from build123d import *

# Parameters (mm, degrees)
F0_R         = 30
F1_DEPTH     = 5
F2_T4_ANGLE  = 130.4484876855
F2_T9_ANGLE  = 130.4484876855
F2_T14_ANGLE = 130.4484876855
F2_T19_ANGLE = 130.4484876855
F2_T24_ANGLE = 130.4484876855
F2_T29_ANGLE = 130.4484876855
F2_T34_ANGLE = 130.4484876855
F2_T39_ANGLE = 130.4484876855
F2_T44_ANGLE = 130.4484876855
F2_T49_ANGLE = 130.4484876855


# Not quite as in the source:
# - a fillet or chamfer that OpenCascade refuses, or shapes differently, is made with other operations: its cross-section is extruded or revolved along the edge and cut away or added


with BuildPart() as f1:
    # F0 (on Top) → F1 (new body)
    with BuildSketch(Plane.XY):
        with BuildLine():
            Line((-40, 12.9967878493), (-24.72135955, 34.0260323341))
            ThreePointArc((-24.72135955, 34.0260323341), (-45.1291822893, 39.7035462239), (-64.2705098312, 30.6303454181))
            Line((-64.2705098312, 30.6303454181), (-40, 12.9967878493))
        make_face()
        Polygon((40, -12.9967878493), (40, 12.9967878493), (24.72135955, 34.0260323341), (0, 42.0584889695), (-24.72135955, 34.0260323341), (-40, 12.9967878493), (-40, -12.9967878493), (-24.72135955, -34.0260323341), (0, -42.0584889695), (24.72135955, -34.0260323341), align=None)
        Circle(F0_R, mode=Mode.SUBTRACT)
        with BuildLine():
            Line((-24.72135955, 34.0260323341), (0, 42.0584889695))
            ThreePointArc((0, 42.0584889695), (-13.1731164802, 58.6471114297), (-33.9918693812, 62.5577278229))
            Line((-33.9918693812, 62.5577278229), (-24.72135955, 34.0260323341))
        make_face()
        with BuildLine():
            Line((0, 42.0584889695), (24.72135955, 34.0260323341))
            ThreePointArc((24.72135955, 34.0260323341), (23.8146320866, 55.1894734115), (9.2705098312, 70.5901844584))
            Line((9.2705098312, 70.5901844584), (0, 42.0584889695))
        make_face()
        with BuildLine():
            Line((24.72135955, 34.0260323341), (40, 12.9967878493))
            ThreePointArc((40, 12.9967878493), (51.7060006259, 30.6513323712), (48.9918693812, 51.6595899029))
            Line((48.9918693812, 51.6595899029), (24.72135955, 34.0260323341))
        make_face()
        with BuildLine():
            Line((70, 12.9967878493), (40, 12.9967878493))
            Line((40, 12.9967878493), (40, -12.9967878493))
            ThreePointArc((40, -12.9967878493), (59.8474343484, -5.5945758344), (70, 12.9967878493))
        make_face()
        with BuildLine():
            Line((64.2705098312, -30.6303454181), (40, -12.9967878493))
            Line((40, -12.9967878493), (24.72135955, -34.0260323341))
            ThreePointArc((24.72135955, -34.0260323341), (45.1291822893, -39.7035462239), (64.2705098312, -30.6303454181))
        make_face()
        with BuildLine():
            Line((33.9918693812, -62.5577278229), (24.72135955, -34.0260323341))
            Line((24.72135955, -34.0260323341), (0, -42.0584889695))
            ThreePointArc((0, -42.0584889695), (13.1731164802, -58.6471114297), (33.9918693812, -62.5577278229))
        make_face()
        with BuildLine():
            Line((-9.2705098312, -70.5901844584), (0, -42.0584889695))
            Line((0, -42.0584889695), (-24.72135955, -34.0260323341))
            ThreePointArc((-24.72135955, -34.0260323341), (-23.8146320866, -55.1894734115), (-9.2705098312, -70.5901844584))
        make_face()
        with BuildLine():
            Line((-48.9918693812, -51.6595899029), (-24.72135955, -34.0260323341))
            Line((-24.72135955, -34.0260323341), (-40, -12.9967878493))
            ThreePointArc((-40, -12.9967878493), (-51.7060006259, -30.6513323712), (-48.9918693812, -51.6595899029))
        make_face()
        with BuildLine():
            Line((-40, -12.9967878493), (-40, 12.9967878493))
            ThreePointArc((-40, 12.9967878493), (-59.8474343484, 5.5945758344), (-70, -12.9967878493))
            Line((-70, -12.9967878493), (-40, -12.9967878493))
        make_face()
    extrude(amount=F1_DEPTH)

    # F2: chamfer of 5 on 10 edges, made by hand


with BuildPart() as f2_tool2:
    # F2_s3 → F2_t4 (revolve)
    with BuildSketch(Plane(origin=(-19.7412033785, -21.6824721062, 0), x_dir=(0, 0, 1), z_dir=(0.6732302342, 0.7394329258, 0))):
        Polygon((0, 1.9388571331), (5, 6.9388571331), (5, 1.9388571331), align=None)
    revolve(axis=Axis((4.103379024, -43.3922083566, 5), (0, 0, 1)), revolution_arc=F2_T4_ANGLE)

    split(bisect_by=Plane(origin=(7.639320225, -10.5146222424, 0), x_dir=(0, 0, 1), z_dir=(0.5877852523, -0.8090169944, 0)), keep=Keep.TOP)


with BuildPart() as f1_1:
    add(f1.part)

    # F2_t1: cut F2_tool2
    add(f2_tool2.part, mode=Mode.SUBTRACT)


with BuildPart() as f2_tool7:
    # F2_s8 → F2_t9 (revolve)
    with BuildSketch(Plane(origin=(-28.7156063599, -5.9379002056, 0), x_dir=(0, 0, 1), z_dir=(0.9792824694, 0.2024990002, 0))):
        Polygon((0, 1.9388571331), (5, 6.9388571331), (5, 1.9388571331), align=None)
    revolve(axis=Axis((-22.1855967717, -37.5169396588, 5), (0, 0, 1)), revolution_arc=F2_T9_ANGLE)

    split(bisect_by=Plane.XZ.offset(12.9967878493), keep=Keep.TOP)


with BuildPart() as f1_2:
    add(f1_1.part)

    # F2_t6: cut F2_tool7
    add(f2_tool7.part, mode=Mode.SUBTRACT)


with BuildPart() as f2_tool12:
    # F2_s13 → F2_t14 (revolve)
    with BuildSketch(Plane(origin=(-26.7216237194, 12.0747477518, 0), x_dir=(0, 0, 1), z_dir=(0.911282086, -0.4117826609, 0))):
        Polygon((0, 1.9388571331), (5, 6.9388571331), (5, 1.9388571331), align=None)
    revolve(axis=Axis((-40.0004286612, -17.3114751652, 5), (0, 0, 1)), revolution_arc=F2_T14_ANGLE)

    split(bisect_by=Plane(origin=(-7.639320225, -10.5146222424, 0), x_dir=(0, 0, 1), z_dir=(-0.5877852523, -0.8090169944, 0)), keep=Keep.TOP)


with BuildPart() as f1_3:
    add(f1_2.part)

    # F2_t11: cut F2_tool12
    add(f2_tool12.part, mode=Mode.SUBTRACT)


with BuildPart() as f2_tool17:
    # F2_s18 → F2_t19 (revolve)
    with BuildSketch(Plane(origin=(-14.5208890526, 25.4752524735, 0), x_dir=(0, 0, 1), z_dir=(0.495202919, -0.8687773415, 0))):
        Polygon((0, 1.9388571331), (5, 6.9388571331), (5, 1.9388571331), align=None)
    revolve(axis=Axis((-42.5364563668, 9.5063844461, 5), (0, 0, 1)), revolution_arc=F2_T19_ANGLE)

    split(bisect_by=Plane(origin=(-12.360679775, -4.0162283177, 0), x_dir=(0, 0, 1), z_dir=(-0.9510565163, -0.3090169944, 0)), keep=Keep.TOP)


with BuildPart() as f1_4:
    add(f1_3.part)

    # F2_t16: cut F2_tool17
    add(f2_tool17.part, mode=Mode.SUBTRACT)


with BuildPart() as f2_tool22:
    # F2_s23 → F2_t24 (revolve)
    with BuildSketch(Plane(origin=(3.2263316853, 29.1450766224, 0), x_dir=(0, 0, 1), z_dir=(-0.1100269317, -0.9939286062, 0))):
        Polygon((0, 1.9388571331), (5, 6.9388571331), (5, 1.9388571331), align=None)
    revolve(axis=Axis((-28.8250035012, 32.6931283091, 5), (0, 0, 1)), revolution_arc=F2_T24_ANGLE)

    split(bisect_by=Plane(origin=(-12.360679775, 4.0162283177, 0), x_dir=(0, 0, 1), z_dir=(-0.9510565163, 0.3090169944, 0)), keep=Keep.TOP)


with BuildPart() as f1_5:
    add(f1_4.part)

    # F2_t21: cut F2_tool22
    add(f2_tool22.part, mode=Mode.SUBTRACT)


with BuildPart() as f2_tool27:
    # F2_s28 → F2_t29 (revolve)
    with BuildSketch(Plane(origin=(19.7412033785, 21.6824721062, 0), x_dir=(0, 0, 1), z_dir=(-0.6732302342, -0.7394329258, 0))):
        Polygon((0, 1.9388571331), (5, 6.9388571331), (5, 1.9388571331), align=None)
    revolve(axis=Axis((-4.103379024, 43.3922083566, 5), (0, 0, 1)), revolution_arc=F2_T29_ANGLE)

    split(bisect_by=Plane(origin=(-7.639320225, 10.5146222424, 0), x_dir=(0, 0, 1), z_dir=(-0.5877852523, 0.8090169944, 0)), keep=Keep.TOP)


with BuildPart() as f1_6:
    add(f1_5.part)

    # F2_t26: cut F2_tool27
    add(f2_tool27.part, mode=Mode.SUBTRACT)


with BuildPart() as f2_tool32:
    # F2_s33 → F2_t34 (revolve)
    with BuildSketch(Plane(origin=(28.7156063599, 5.9379002056, 0), x_dir=(0, 0, 1), z_dir=(-0.9792824694, -0.2024990002, 0))):
        Polygon((0, 1.9388571331), (5, 6.9388571331), (5, 1.9388571331), align=None)
    revolve(axis=Axis((22.1855967717, 37.5169396588, 5), (0, 0, 1)), revolution_arc=F2_T34_ANGLE)

    split(bisect_by=Plane.XZ.offset(-12.9967878493), keep=Keep.BOTTOM)


with BuildPart() as f1_7:
    add(f1_6.part)

    # F2_t31: cut F2_tool32
    add(f2_tool32.part, mode=Mode.SUBTRACT)


with BuildPart() as f2_tool37:
    # F2_s38 → F2_t39 (revolve)
    with BuildSketch(Plane(origin=(26.7216237194, -12.0747477518, 0), x_dir=(0, 0, 1), z_dir=(-0.911282086, 0.4117826609, 0))):
        Polygon((0, 1.9388571331), (5, 6.9388571331), (5, 1.9388571331), align=None)
    revolve(axis=Axis((40.0004286612, 17.3114751652, 5), (0, 0, 1)), revolution_arc=F2_T39_ANGLE)

    split(bisect_by=Plane(origin=(7.639320225, 10.5146222424, 0), x_dir=(0, 0, 1), z_dir=(0.5877852523, 0.8090169944, 0)), keep=Keep.TOP)


with BuildPart() as f1_8:
    add(f1_7.part)

    # F2_t36: cut F2_tool37
    add(f2_tool37.part, mode=Mode.SUBTRACT)


with BuildPart() as f2_tool42:
    # F2_s43 → F2_t44 (revolve)
    with BuildSketch(Plane(origin=(14.5208890526, -25.4752524735, 0), x_dir=(0, 0, 1), z_dir=(-0.495202919, 0.8687773415, 0))):
        Polygon((0, 1.9388571331), (5, 6.9388571331), (5, 1.9388571331), align=None)
    revolve(axis=Axis((42.5364563668, -9.5063844461, 5), (0, 0, 1)), revolution_arc=F2_T44_ANGLE)

    split(bisect_by=Plane(origin=(12.360679775, 4.0162283177, 0), x_dir=(0, 0, 1), z_dir=(0.9510565163, 0.3090169944, 0)), keep=Keep.TOP)


with BuildPart() as f1_9:
    add(f1_8.part)

    # F2_t41: cut F2_tool42
    add(f2_tool42.part, mode=Mode.SUBTRACT)


with BuildPart() as f2_tool47:
    # F2_s48 → F2_t49 (revolve)
    with BuildSketch(Plane(origin=(-3.2263316853, -29.1450766224, 0), x_dir=(0, 0, 1), z_dir=(0.1100269317, 0.9939286062, 0))):
        Polygon((0, 1.9388571331), (5, 6.9388571331), (5, 1.9388571331), align=None)
    revolve(axis=Axis((28.8250035012, -32.6931283091, 5), (0, 0, 1)), revolution_arc=F2_T49_ANGLE)

    split(bisect_by=Plane(origin=(12.360679775, -4.0162283177, 0), x_dir=(0, 0, 1), z_dir=(0.9510565163, -0.3090169944, 0)), keep=Keep.TOP)


with BuildPart() as f1_10:
    add(f1_9.part)

    # F2_t46: cut F2_tool47
    add(f2_tool47.part, mode=Mode.SUBTRACT)


solid = f1_10.part
Source: CAD feature listing. Evaluate the final solid. Frame: model axes, mm. Coordinates: 2 decimals unless noted, no trailing zeros. Loops run counter-clockwise (first coordinate to the right, second up) from the corner with the lowest first, then second, coordinate; pieces in that order, holes last. Notation, with made-up numbers: (82, -2.75) -> (109, -2.75) arc R20 cw to (109, 4.25) -> close; hole circle Ø1 at (-12, 89.5). An arc over 180 degrees is marked (long way). Answer in a Markdown table with one row per item. Add a question column.
Q1. Section A-A on z = 1.65. Return the cut outline in (x, y) (3 decimals), and give its area (3 significant figures).
Q2. Ray query, line 1 along X through (y, z) = (26.5, 4.05); line 2 along Y through (x, z) = (-42, 2.65); line 3 along Y through (x, z) = (-11.5, 1.6). Return the intervals inside material, ascending.
Q3. Contact query for flat-ended pins moving along their axis: pin 1 Ø2 at (x, y) = (28, -6.5) entering from -Z; pin 2 Ø1 at (y, z) = (12.5, 1) entering from +X; pin 3 Ø3 at (y, z) = (1, 3) entering from +X. Output: stop coordinate, or through.
Q4. Pull-direction query (Y, two-part tool) for faces 1 (the face through (-1, -30.4, 0)), 2 (the face through (-29.97, 1.32, 2.46)); classes: pulls with the +Y half, pulls with the -Y half, needs draft (parallel to the pull), parting line crosses it, or undercut.
Q5. Section B-B on y = -46.5. Give the number of separate pieces and of enclosed holes in the cut face, and give its area (3 significant figures).
Computed values:
| question | item | result |
|---|---|---|
| 1 | outline | (-68.332, -12.997) -> (-37.02, -12.997) arc R28.658 ccw to (-47.642, -50.679) -> (-22.31, -32.274) arc R28.658 ccw to (-8.755, -69.004) -> (0.921, -39.224) arc R28.658 ccw to (33.476, -60.971) -> (23.8, -31.192) arc R28.658 ccw to (62.921, -29.65) -> (37.589, -11.245) arc R28.658 ccw to (68.332, 12.997) -> (37.02, 12.997) arc R28.658 ccw to (47.642, 50.679) -> (22.31, 32.274) arc R28.658 ccw to (8.755, 69.004) -> (-0.921, 39.224) arc R28.658 ccw to (-33.476, 60.971) -> (-23.8, 31.192) arc R28.658 ccw to (-62.921, 29.65) -> (-37.589, 11.245) arc R28.658 ccw to start; hole circle Ø60 at (0, 0) |
| 1 | area | 7,570 mm^2 |
| 2 | line 1 | x = -58.59 to -22.52, -22.28 to -14.06, 14.06 to 46.02 |
| 2 | line 2 | y = -46.58 to -18.22, -13 to 10.27, 14.45 to 37.16 |
| 2 | line 3 | y = -67.49 to -27.71, 27.71 to 55.58 |
| 3 | pin 1 | passes through |
| 3 | pin 2 | stops at x = 69.42 |
| 3 | pin 3 | stops at x = 64.01 |
| 4 | face 1 | needs draft |
| 4 | face 2 | undercut |
| 5 | separate pieces | 3 |
| 5 | enclosed holes | 0 |
| 5 | area | 264 mm^2 |
